Verification items for this drawing (mm, ordinates from the low corner). A direction names the side the tool comes from. Give positions to 0.01 mm unless a question says otherwise; leave off trailing zeros. Loops run counter-clockwise (first coordinate to the right, second up) from the corner with the lowest first, then second, coordinate; pieces in that order, holes last. Notation, with made-up numbers: M -14,67.25 L 37,67.25 A14 ccw 37,89.25 Z; hole C -3.5,46 d1. An arc over 180 degrees is marked long. Answer in a Markdown table with one row per item.
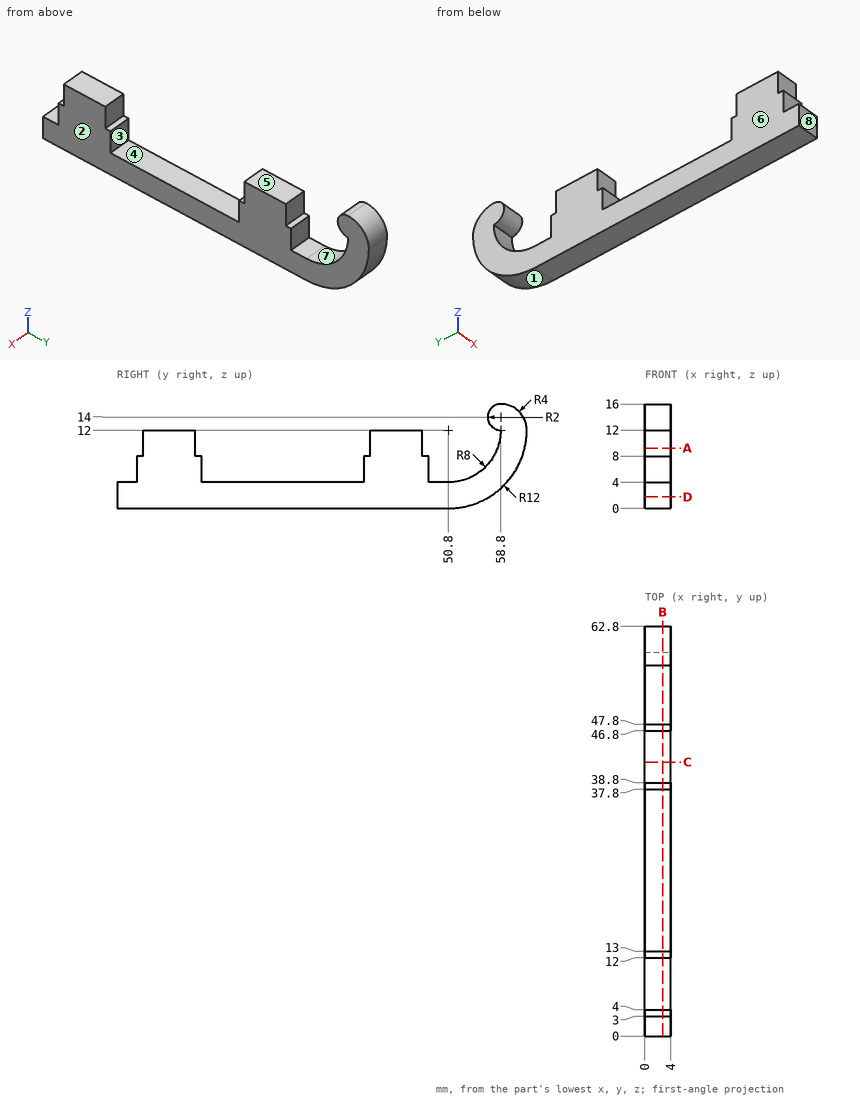
Item 1: Scan lines: L1, parallel to Y at x = 1.1, z = 11.25; L2, parallel to Y at x = 0.7, z = 10.5; L3, parallel to Z at x = 2.5, y = 50. Record each from-to range of solid material in increasing order. Write a range as [from, to].
Reported:
| item | result |
|---|---|
| L1 | y = [4, 12], [38.8, 46.8], [58.76, 62.78] |
| L2 | y = [4, 12], [38.8, 46.8], [58.66, 62.71] |
| L3 | z = [0, 4] |
Item 2: Sectioned sample at B-B (x = 2.75). Record the cut outline in (y, z).
Reported:
| item | result |
|---|---|
| outline | M 0,0 L 50.8,0 A12 ccw 62.8,12 A4 ccw 58.8,16 A2 ccw 58.8,12 A8 cw 50.8,4 L 47.8,4 L 47.8,8 L 46.8,8 L 46.8,12 L 38.8,12 L 38.8,8 L 37.8,8 L 37.8,4 L 13,4 L 13,8 L 12,8 L 12,12 L 4,12 L 4,8 L 3,8 L 3,4 L 0,4 Z |
Item 3: Sectioned sample at A-A (z = 9.25). Record the cut outline in (x, y).
Reported:
| item | result |
|---|---|
| outline | M 0,4 L 4,4 L 4,12 L 0,12 Z; M 0,38.8 L 4,38.8 L 4,46.8 L 0,46.8 Z; M 0,58.31 L 4,58.31 L 4,62.48 L 0,62.48 Z |
Item 4: Tool access check on the marked faces 4, 5, 6, 7 and 8. Record the directions out of +Z, -Z, +X, -X, +Y, -Y that give a thin tool (end or side, any length) a straight path to the whole face; none if there is none.
Reported:
| item | result |
|---|---|
| face 4 | +Z, +X, -X |
| face 5 | +Z, +X, -X, -Y |
| face 6 | +Z, -Z, -X, +Y, -Y |
| face 7 | +X, -X |
| face 8 | +Z, -Z, +X, -X, -Y |
Item 5: Sectioned sample at C-C (y = 42). Record the cut outline in (x, z).
Reported:
| item | result |
|---|---|
| outline | M 0,0 L 4,0 L 4,12 L 0,12 Z |
Item 6: Sectioned sample at D-D (z = 1.75). Record the cut outline in (x, y), and give its area (3 significant figures).
Reported:
| item | result |
|---|---|
| outline | M 0,0 L 4,0 L 4,57.04 L 0,57.04 Z |
| area | 228 mm^2 |
Item 7: Go/stop test with flat-tipped pins: pin 1 (0.5 mm diameter, centred on x = 2, y = 38.5, fed in from +Z); pin 2 (2 mm diameter, centred on x = 2.5, z = 9.5, fed in from +Y); pin 3 (1.2 mm diameter, centred on x = 1.5, z = 5.5, fed in from -Y); pin 4 (6 mm diameter, centred on y = 25.5, z = 9, fed in from -X). Record where each tip stops, or that it passes through.
Reported:
| item | result |
|---|---|
| pin 1 | stops at z = 8 |
| pin 2 | stops at y = 62.71 |
| pin 3 | stops at y = 3 |
| pin 4 | passes through |
Item 8: Release check for a two-part mould opening along Y. For the marked faces 1, 2 and 3 record: released by +Y, released by -Y, zero draft, split by the parting line, or undercut.
Reported:
| item | result |
|---|---|
| face 1 | released by +Y |
| face 2 | zero draft |
| face 3 | undercut |
